Build history of the part. All positions in model axes, mm. Round coordinates to 2 decimals unless told otherwise and drop trailing zeros. Loops run counter-clockwise (first coordinate to the right, second up) from the corner with the lowest first, then second, coordinate; pieces in that order, holes last.
Autodesk Inventor part; units mm, degrees
ref_plane "YZ Plane" through (0, 0, 0) normal (1, 0, 0) x (0, 1, 0)
ref_plane "XZ Plane" through (0, 0, 0) normal (0, 1, 0) x (-1, 0, 0)
ref_plane "XY Plane" through (0, 0, 0) normal (0, 0, 1) x (1, 0, 0)
sketch "スケッチ1" plane through (0, 0, 0) normal (0, 0, 1) x (1, 0, 0)
  circle A0 centre (0, 0) radius 2
  dimension "d0" = 4
extrude "押し出し1" add sketch "スケッチ1" along normal blind 6
sketch "スケッチ2" plane through (0, 0, 6) normal (0, 0, 1) x (1, 0, 0)
  circle A0 centre (0, 0) radius 2
  circle A1 centre (0, 0) radius 4
  dimension "d3" = 8
extrude "押し出し2" add sketch "スケッチ2" along normal blind 2.3 contours A0 | A1
thread "ねじ1"
chamfer "面取り1" distance 2 angle 45 1 edges at (-4, 0, 6)
sketch "スケッチ4" plane through (0, 0, 0) normal (0, 0, -1) x (-1, 0, 0)
  circle A0 centre (0, 0) radius 2
extrude "押し出し4" add sketch "スケッチ4" along normal blind 6.7
properties part number "SB　M4 15mm 皿ネジ" material "Stainless Steel, 440C"
(1) Pin check, flat tips, straight feed: P1, Ø2, axis at y = -2.5, z = -1, coming from the -X side; P2, Ø1, axis at x = 0, z = -4, coming from the +Y side; P3, Ø4, axis at x = 3, z = -5, coming from the +Y side. Stop position of each tip, or through.
Responses:
P1: stops at x = -1.32
P2: stops at y = 2
P3: stops at y = 1.73
(2) Slice it at D-D on z = 6.5. List the corners of the cut face in (x, y), plus the area to 3 significant figures.
Responses:
outline: circle Ø5 at (0, 0)
area: 19.6 mm2
(3) Slice it at C-C on z = 5. List the corners of the cut face in (x, y).
Responses:
outline: circle Ø4 at (0, 0)
(4) Probe line 1 (Y direction, x = 1.5, z = 6.5); line 2 (X direction, y = -0.5, z = 3.25); line 3 (Y direction, x = 0.75, z = 4.75). List the from-to ranges inside material, lowest first.
Responses:
line 1: y = -2 to 2
line 2: x = -1.94 to 1.94
line 3: y = -1.85 to 1.85
